Geometry: see drawing. Coordinates: mm, zero at the bounding-box minimum. A direction names the side the tool comes from. Coordinates: 2 decimals unless noted, no trailing zeros. Order: outer loops, then holes, each group sorted by start corner. A loop starts at its lowest first (then second) coordinate and runs counter-clockwise, first axis right, second up. Notation, with made-up numbers: M 58.5,35 L 81.5,35 A7 ccw 81.5,42 Z; hole C 13,23.5 d3. An arc over 180 degrees is marked long. One line per item, written item: value.
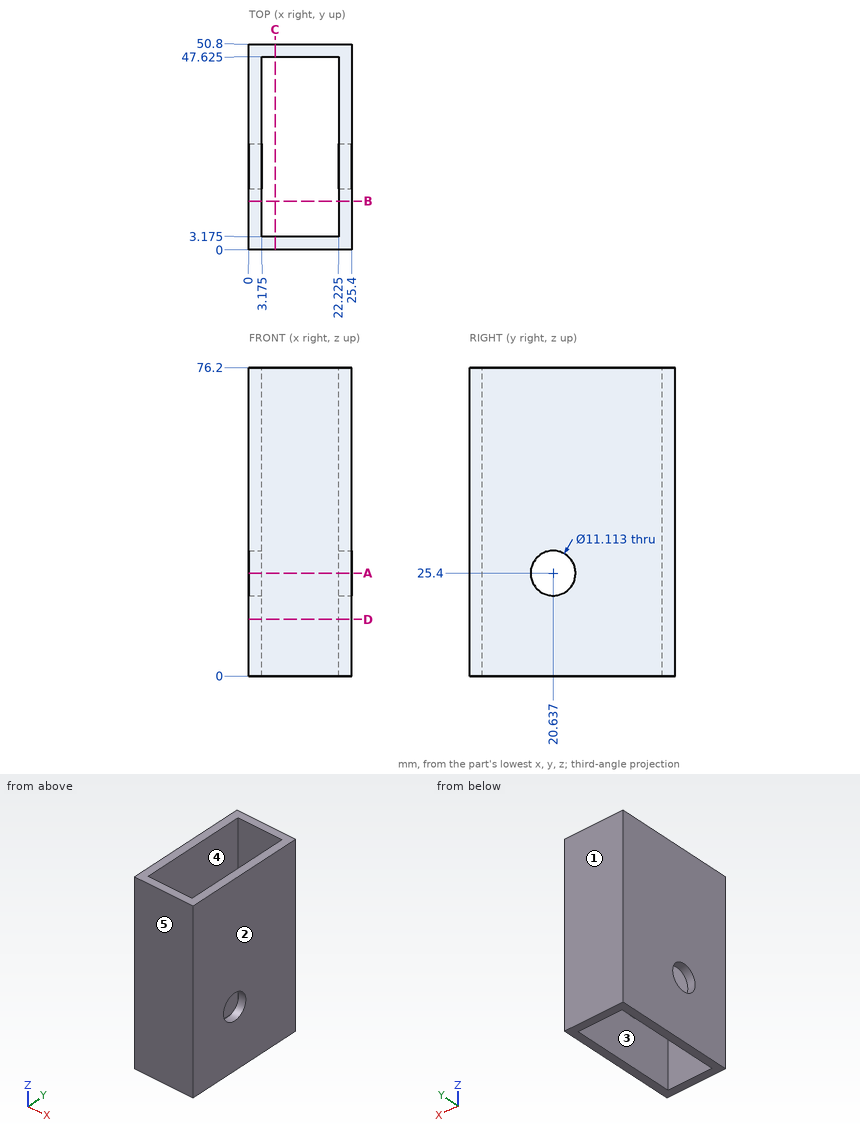
(1) Ray query, line 1 (Y direction, x = 17.5, z = 32.5) (1 decimal); line 2 (X direction, y = 43.5, z = 19) (1 decimal); line 3 (Y direction, x = 24.2, z = 25.4). Return the intervals inside material, ascending. Write a range as from..to.
Data:
line 1: y = 0..3.2, 47.6..50.8
line 2: x = 0..3.2, 22.2..25.4
line 3: y = 0..15.08, 26.19..50.8
(2) Draft query along X for the marked faces 1, 2 and 3. Return one class per face: released by +X, released by -X, zero draft, split by the parting line, or undercut.
Data:
face 1: zero draft
face 2: released by +X
face 3: undercut
(3) Cut plane B-B on y = 12. Output: boundary loops of the cut face in (x, z) (1 decimal).
Data:
outline: M 0,0 L 3.2,0 L 3.2,76.2 L 0,76.2 Z; M 22.2,0 L 25.4,0 L 25.4,76.2 L 22.2,76.2 Z
(4) Cut plane A-A on z = 25.4. Output: boundary loops of the cut face in (x, y) (1 decimal).
Data:
outline: M 0,0 L 25.4,0 L 25.4,15.1 L 22.2,15.1 L 22.2,3.2 L 3.2,3.2 L 3.2,15.1 L 0,15.1 Z; M 0,26.2 L 3.2,26.2 L 3.2,47.6 L 22.2,47.6 L 22.2,26.2 L 25.4,26.2 L 25.4,50.8 L 0,50.8 Z
(5) Cut plane D-D on z = 14. Output: boundary loops of the cut face in (x, y) (1 decimal).
Data:
outline: M 0,0 L 25.4,0 L 25.4,50.8 L 0,50.8 Z; hole M 3.2,3.2 L 22.2,3.2 L 22.2,47.6 L 3.2,47.6 Z
(6) Cut plane C-C on x = 6.5. Output: boundary loops of the cut face in (y, z) (1 decimal), plus the area to 3 significant figures.
Data:
outline: M 0,0 L 3.2,0 L 3.2,76.2 L 0,76.2 Z; M 47.6,0 L 50.8,0 L 50.8,76.2 L 47.6,76.2 Z
area: 484 mm2
(7) Access query for the marked faces 4 and 5. Directions: +Z, -Z, +X, -X, +Y, -Y. A direction counts if a zero-diameter tool reaches every point of the face in a straight line with its end or side. Return the directions, or none.
Data:
face 4: +Z, -Z
face 5: +Z, -Z, +X, -X, -Y
